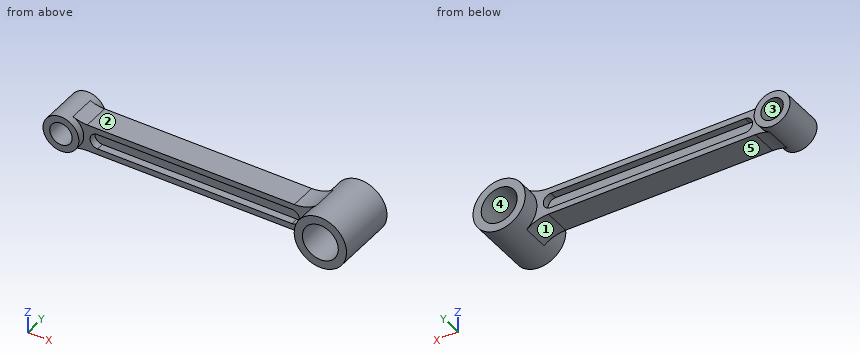
from build123d import *

# Parameters (mm, degrees)
SKETCH1_R           = 12
SKETCH1_R_2         = 7.5
BOSS_EXTRUDE1_DEPTH = 14
SKETCH1_3_R         = 17.5
SKETCH1_3_R_2       = 12
BOSS_EXTRUDE2_DEPTH = 21
BOSS_EXTRUDE3_DEPTH = 9
CUT_EXTRUDE1_START  = 9
CUT_EXTRUDE1_DEPTH  = 5


with BuildPart() as part:
    # Sketch1 → Boss-Extrude1 (new, symmetric)
    with BuildSketch(Plane(origin=(0, 0, 0), x_dir=(1, 0, 0), z_dir=(0, 1, 0))):
        with Locations(Location((-54.333170882, 0, 0), (0, 0, 270))):
            Circle(SKETCH1_R)
        with Locations(Location((-54.333170882, 0, 0), (0, 0, 270))):
            Circle(SKETCH1_R_2, mode=Mode.SUBTRACT)
    extrude(amount=BOSS_EXTRUDE1_DEPTH, both=True)



with BuildPart() as body_2:
    # Sketch1_3 → Boss-Extrude2 (new, symmetric)
    with BuildSketch(Plane(origin=(0, 0, 0), x_dir=(1, 0, 0), z_dir=(0, 1, 0))):
        with Locations(Location((123.666829118, 0, 0), (0, 0, 90))):
            Circle(SKETCH1_3_R)
        with Locations(Location((123.666829118, 0, 0), (0, 0, 90))):
            Circle(SKETCH1_3_R_2, mode=Mode.SUBTRACT)
    extrude(amount=BOSS_EXTRUDE2_DEPTH, both=True)


with BuildPart() as part_1:
    add(part.part)

    add(body_2.part)  # Boss-Extrude3 merges body 2
    # Sketch1_4 → Boss-Extrude3 (add, symmetric)
    with BuildSketch(Plane(origin=(0, 0, 0), x_dir=(1, 0, 0), z_dir=(0, 1, 0))):
        with BuildLine():
            Line((98.502370054, 9), (-39.945676312, 9))
            ThreePointArc((-39.945676312, 9), (-44.844655798, 9.505319751), (-49.537339359, 11))
            ThreePointArc((-49.537339359, 11), (-42.333170882, 0), (-49.537339359, -11))
            ThreePointArc((-49.537339359, -11), (-44.844655798, -9.505319751), (-39.945676312, -9))
            Line((-39.945676312, -9), (98.502370054, -9))
            ThreePointArc((98.502370054, -9), (106.182731491, -10.26210106), (113.055310235, -13.915662651))
            ThreePointArc((113.055310235, -13.915662651), (106.166829118, 0), (113.055310235, 13.915662651))
            ThreePointArc((113.055310235, 13.915662651), (106.182731491, 10.26210106), (98.502370054, 9))
        make_face()
    extrude(amount=BOSS_EXTRUDE3_DEPTH, both=True)

    # Sketch1_5 → Cut-Extrude1 (cut)
    with BuildSketch(Plane(origin=(0, 0, 0), x_dir=(1, 0, 0), z_dir=(0, 1, 0)).offset(CUT_EXTRUDE1_START)):
        with BuildLine():
            Line((-33.083170882, 5), (96.916829118, 5))
            ThreePointArc((96.916829118, 5), (101.916829118, 0), (96.916829118, -5))
            Line((96.916829118, -5), (-33.083170882, -5))
            ThreePointArc((-33.083170882, -5), (-38.083170882, 0), (-33.083170882, 5))
        make_face()
    cut_extrude1 = extrude(amount=-CUT_EXTRUDE1_DEPTH, mode=Mode.SUBTRACT)

    # Mirror1: Cut-Extrude1 across plane
    add(cut_extrude1.mirror(Plane.ZX), mode=Mode.SUBTRACT)


solid = part_1.part
Work out the finished part from the listing and answer in its coordinate system (mm). Face numbers are marked on the shaded views. A direction names the side the tool comes from. Round coordinates to 2 decimals unless told otherwise and drop trailing zeros. Write each loop counter-clockwise with the first axis right and the second up, starting at its lowest first coordinate (ties: lowest second). Pieces come first, ordered by that corner, then holes. Notation, with made-up numbers: (-29, -36) -> (27, -36) arc R19 cw to (27, -27) -> close; hole circle Ø5 at (-9, 77). An arc over 180 degrees is marked (long way). Answer as CSV lines item,"result". Start each with the question number.
(1) The part is cut by section D-D, the plane y = 11.5. Give the vertices of the cut face in (x, z).
(2) The part is cut by section A-A, the plane z = 0. Give the vertices of the cut face in (x, y), then the cut area to 3 significant figures.
(3) Find the intervals of material crossed by probe 1 along X at (y, z) = (-5, 0); probe 2 along X at (y, z) = (2, 0); probe 3 along Z at (x, y) = (-23, -8), in increasing order.
(4) The part is cut by section C-C, the plane y = 0. Give the vertices of the cut face in (x, z), then the cut area to 3 significant figures.
(5) A tool of negligible diameter and unlimited length cuts with its end or side. For the marked faces 4 and 5, from which of +Z, -Z, +X, -X, +Y, -Y can it reach the whole face along a straight path? Write none if from no direction.
(6) The mould has two halves that part along Z. Classify the marked faces 1, 2 and 3: +Z half, -Z half, draft (parallel to the pull), parting line (faces both ways), or undercut.
(7) Each of these flat-tipped pins is pushed along its axis until it touches: pin 1 (19 mm diameter, centred on x = 123.67, z = 0, fed in from -Y); pin 2 (2.5 mm diameter, centred on x = 2, y = 7.5, fed in from -Z); pin 3 (19.5 mm diameter, centred on x = -54.33, z = 0, fed in from -Y); pin 4 (2.5 mm diameter, centred on x = 16, y = 6, fed in from +Z). Where does it stop, or does it pass through?
(8) The part is cut by section B-B, the plane x = -30.5. Give the vertices of the cut face in (y, z), then the cut area to 3 significant figures.
Output values:
1,outline,"circle Ø24 at (-54.33, 0); circle Ø35 at (123.67, 0); hole circle Ø15 at (-54.33, 0); hole circle Ø24 at (123.67, 0)"
2,outline,"(-66.33, -14) -> (-61.83, -14) -> (-61.83, 14) -> (-66.33, 14) -> close; (-46.83, -14) -> (-42.33, -14) -> (-42.33, -9) -> (-38.08, -9) -> (-38.08, -4) -> (101.92, -4) -> (101.92, -9) -> (106.17, -9) -> (106.17, -21) -> (111.67, -21) -> (111.67, 21) -> (106.17, 21) -> (106.17, 9) -> (101.92, 9) -> (101.92, 4) -> (-38.08, 4) -> (-38.08, 9) -> (-42.33, 9) -> (-42.33, 14) -> (-46.83, 14) -> close; (135.67, -21) -> (141.17, -21) -> (141.17, 21) -> (135.67, 21) -> close"
2,area,"1,990 mm²"
3,probe 1,"x = -66.33 to -61.83, -46.83 to -38.08, 101.92 to 111.67, 135.67 to 141.17"
3,probe 2,"x = -66.33 to -61.83, -46.83 to 111.67, 135.67 to 141.17"
3,probe 3,"z = -9 to -5, 5 to 9"
4,outline,"(-49.54, -11) arc R24 cw to (-39.95, -9) -> (98.5, -9) arc R24 cw to (113.06, -13.92) arc R17.5 ccw (long way) to (113.06, 13.92) arc R24 cw to (98.5, 9) -> (-39.95, 9) arc R24 cw to (-49.54, 11) arc R12 ccw (long way) to start; hole circle Ø15 at (-54.33, 0); hole circle Ø24 at (123.67, 0)"
4,area,"3,520 mm²"
5,face 4,"+Y, -Y"
5,face 5,"-Z, +Y, -Y"
6,face 1,"-Z half"
6,face 2,"+Z half"
6,face 3,"undercut"
7,pin 1,"passes through"
7,pin 2,"stops at z = -9"
7,pin 3,"stops at y = -14"
7,pin 4,"stops at z = 9"
8,outline,"(-9, -9) -> (9, -9) -> (9, -5) -> (4, -5) -> (4, 5) -> (9, 5) -> (9, 9) -> (-9, 9) -> (-9, 5) -> (-4, 5) -> (-4, -5) -> (-9, -5) -> close"
8,area,"224 mm²"
